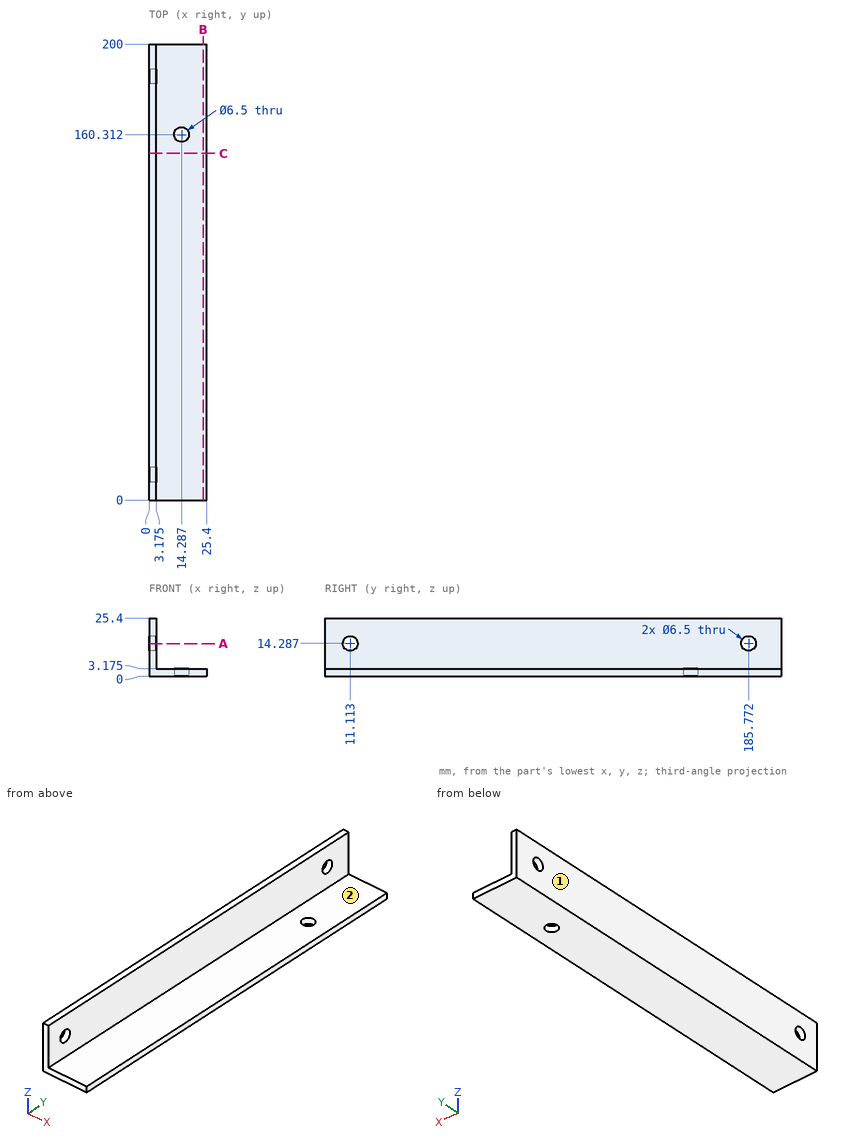
Design review of the part shown in the three views and the two pictorial views. Dimensions are in mm from the part's minimum x, y and z. A direction names the side the tool comes from. Round coordinates to 2 decimals unless told otherwise and drop trailing zeros. Loops run counter-clockwise (first coordinate to the right, second up) from the corner with the lowest first, then second, coordinate; pieces in that order, holes last.
1) Tool access review of the marked faces 1 and 2: name each direction out of +Z, -Z, +X, -X, +Y, -Y from which nothing blocks a thin tool from reaching the whole face with its end or side.
Values follow:
face 1: +Z, -Z, -X, +Y, -Y
face 2: +Z, +X, +Y, -Y
2) Consider section A-A on z = 14.25. State the section outline as (x, y) points (3 decimals).
Values follow:
outline: (0, 0) - (3.175, 0) - (3.175, 7.863) - (0, 7.863) - close; (0, 14.363) - (3.175, 14.363) - (3.175, 182.522) - (0, 182.522) - close; (0, 189.022) - (3.175, 189.022) - (3.175, 200) - (0, 200) - close
3) Wall thickness on line 1 along X through (y, z) = (27.5, 6.75) (3 decimals): over which ranges is the line inside the solid? List them lowest first.
Values follow:
line 1: x = 0 to 3.175
4) Clearance check with flat-ended pins moving along their axes: P1, Ø6, axis at x = 9, y = 36.5, coming from the +Z side (3 decimals); P2, Ø10.5, axis at y = 185.772, z = 14.287, coming from the +X side (3 decimals). State where each tip first meets the part, or that it passes through.
Values follow:
P1: stops at z = 3.175
P2: stops at x = 3.175
5) Consider section B-B on x = 23.75. State the section outline as (y, z) points (3 decimals).
Values follow:
outline: (0, 0) - (200, 0) - (200, 3.175) - (0, 3.175) - close
6) Consider section C-C on y = 152. State the section outline as (x, z) points (3 decimals).
Values follow:
outline: (0, 0) - (25.4, 0) - (25.4, 3.175) - (3.175, 3.175) - (3.175, 25.4) - (0, 25.4) - close
